Could you check a few things on this model? Use its own coordinates, in mm. Give positions to 0.01 mm unless a question says otherwise; leave off trailing zeros. Loops run counter-clockwise (first coordinate to the right, second up) from the corner with the lowest first, then second, coordinate; pieces in that order, holes last. Notation, with made-up numbers: (-25, 71.25) -> (34, 71.25) arc R30 cw to (34, 102.25) -> close; hole circle Ø2 at (-3, 14). An arc over 180 degrees is marked (long way). Put each result on its own line as item: value.
```python
from build123d import *

# Parameters (mm, degrees)
SKETCH1_W           = 50
SKETCH1_H           = 30
BOSS_EXTRUDE1_DEPTH = 10
SKETCH2_W           = 135
SKETCH2_H           = 10
SKETCH2_W_2         = 75
BOSS_EXTRUDE3_DEPTH = 10
FILLET1_R           = 5
FILLET2_R           = 5


with BuildPart() as part:
    # Sketch1 → Boss-Extrude1 (new body)
    with BuildSketch(Plane(origin=(0, 0, 0), x_dir=(1, 0, 0), z_dir=(0, 1, 0))):
        Rectangle(SKETCH1_W, SKETCH1_H)
        with BuildLine():
            Line((-4, 3), (-4, -3))
            ThreePointArc((-4, -3), (0, -5), (4, -3))
            Line((4, -3), (4, 3))
            ThreePointArc((4, 3), (0, 5), (-4, 3))
        make_face(mode=Mode.SUBTRACT)
    extrude(amount=BOSS_EXTRUDE1_DEPTH)

    # Sketch2 → Boss-Extrude3 (add)
    with BuildSketch(Plane.XZ):
        with Locations((-92.5, 0)):
            Rectangle(SKETCH2_W, SKETCH2_H)
        with Locations((62.5, 0)):
            Rectangle(SKETCH2_W_2, SKETCH2_H)
    extrude(amount=-BOSS_EXTRUDE3_DEPTH)

    # Fillet1
    fillet1_edges = [part.edges().sort_by_distance(p)[0] for p in [
        (-25, 5, 5),
        (-25, 5, -5),
        (25, 5, -5),
        (25, 5, 5),
    ]]
    fillet(fillet1_edges, radius=FILLET1_R)

    # Fillet2
    fillet2_edges = [part.edges().sort_by_distance(p)[0] for p in [
        (25, 5, 15),
        (-25, 5, 15),
        (-25, 5, -15),
        (25, 5, -15),
    ]]
    fillet(fillet2_edges, radius=FILLET2_R - 0.0001)  # a hair under: the kernel refuses the full size


solid = part.part
```
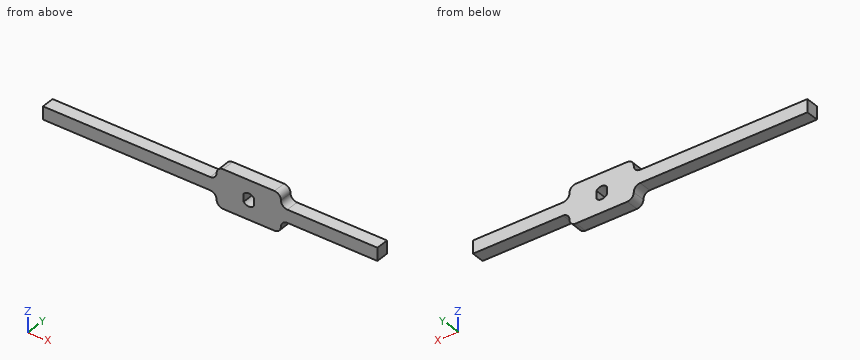
1. If we section it at C-C (x = -108.5): List the corners of the cut face in (y, z) for me, then the cut area to 3 significant figures.
Recorded:
outline: (0, -5) -> (10, -5) -> (10, 5) -> (0, 5) -> close
area: 100 mm^2
2. If we section it at D-D (z = -12.75): List the corners of the cut face in (x, y) for me.
Recorded:
outline: (-24.18, 0) -> (24.18, 0) -> (24.18, 10) -> (-24.18, 10) -> close
3. I'm going to push flat-ended pins straight in: pin 1 (4 mm diameter, centred on y = 6, z = 10, fed in from +X); pin 2 (4 mm diameter, centred on x = -103.5, y = 7, fed in from +Z); pin 3 (1 mm diameter, centred on x = -81, y = 3, fed in from -Z). Where does each tip first touch, or does it pass through?
Recorded:
pin 1: stops at x = 25.42
pin 2: stops at z = 5
pin 3: stops at z = -5
4. If we section it at A-A (z = -0.75): List the corners of the cut face in (x, y) for me.
Recorded:
outline: (-160, 0) -> (-4, 0) -> (-4, 10) -> (-160, 10) -> close; (4, 0) -> (100, 0) -> (100, 10) -> (4, 10) -> close
5. I need wall thicknesses on line 1 (X direction, y = 3, z = 1.75); line 2 (X direction, y = 3.25, z = 3.25); line 3 (X direction, y = 6, z = 10). Which ranges of each line are inside material? Lowest first, please.
Recorded:
line 1: x = -160 to -4, 4 to 100
line 2: x = -160 to -3.8, 3.8 to 100
line 3: x = -25 to 25
